Could you check a few things on this model? Use its own coordinates, in mm. Coordinates: 2 decimals unless noted, no trailing zeros. Write each loop counter-clockwise with the first axis right and the second up, starting at its lowest first coordinate (ties: lowest second). Pieces come first, ordered by that corner, then holes.
```python
from build123d import *

# Parameters (mm, degrees)
F0_W           = 80
F0_H           = 44
F1_DEPTH       = 4
F3_D           = 2.5
F3_DEPTH       = 10
F3_CSINK_D     = 5
F3_CSINK_ANGLE = 81
F5_D           = 4
F5_DEPTH       = 10
F7_D           = 5
F7_DEPTH       = 10
F8_W           = 49.9
F8_H           = 3
F8_W_2         = 2
F8_H_2         = 26
F9_DEPTH       = 1


with BuildPart() as f1:
    # F0 (on Top) → F1 (new body)
    with BuildSketch(Plane.XY):
        Rectangle(F0_W, F0_H)
    extrude(amount=F1_DEPTH)

    # F3
    with Locations(Plane.XY.offset(4)):
        with Locations((-35.7, -17.7), (-35.7, 17.7), (35.7, 17.7), (35.7, -17.7)):
            CounterSinkHole(F3_D / 2, F3_CSINK_D / 2, depth=F3_DEPTH, counter_sink_angle=F3_CSINK_ANGLE)

    # F5
    with Locations(Plane.XY.offset(4)):
        with Locations((-18.5, 15), (-4.5, 15), (9.5, 15), (23.5, 15), (-25.5, 7), (-11.5, 7), (2.5, 7), (16.5, 7), (30.5, 7), (-18.5, 0), (-4.5, 0), (9.5, 0), (23.5, 0), (-25.5, -8), (-11.5, -8), (2.5, -8), (16.5, -8), (30.5, -8), (-18.5, -15), (-4.5, -15), (9.5, -15), (23.5, -15)):
            Hole(F5_D / 2, depth=F5_DEPTH)

    # F7
    with Locations(Plane.XY.offset(4)):
        with Locations((31.5, -0.75)):
            Hole(F7_D / 2, depth=F7_DEPTH)

    # F8 (on face) → F9 (join)
    with BuildSketch(Plane(origin=(0, 0, 0), x_dir=(1, 0, 0), z_dir=(0, 0, -1))):
        with Locations((2.5, 20.5)):
            Rectangle(F8_W, F8_H)
        with Locations((2.5, -20.5)):
            Rectangle(F8_W, F8_H)
        with Locations((35.93, 0)):
            Rectangle(F8_W_2, F8_H_2)
        with Locations((-35.93, 0)):
            Rectangle(F8_W_2, F8_H_2)
    extrude(amount=F9_DEPTH)


solid = f1.part
```
1. I want a section at B-B on y = 7. Give the number of separate pieces and of enclosed holes in the cut face, plus the area to 3 significant figures.
Verdict:
separate pieces: 6
enclosed holes: 0
area: 244 mm2
2. Please list where these lines run through material, in increasing order: line 1 along Y through (x, z) = (-35.7, 1); line 2 along Y through (x, z) = (23.5, 1.85); line 3 along Y through (x, z) = (16.5, 3.1).
Verdict:
line 1: y = -22 to -18.95, -16.45 to 16.45, 18.95 to 22
line 2: y = -22 to -17, -13 to -2, 2 to 13, 17 to 22
line 3: y = -22 to -10, -6 to 5, 9 to 22
3. I want a section at D-D on y = -12. Please give me the cut outline in (x, z), plus the area to 3 significant figures.
Verdict:
outline: (-40, 0) - (-36.93, 0) - (-36.93, -1) - (-34.93, -1) - (-34.93, 0) - (34.93, 0) - (34.93, -1) - (36.93, -1) - (36.93, 0) - (40, 0) - (40, 4) - (-40, 4) - close
area: 324 mm2
4. I want a section at A-A on x = 35.7. Please give me the cut outline in (y, z), plus the area to 3 significant figures.
Verdict:
outline: (-22, 0) - (-18.95, 0) - (-18.95, 2.54) - (-20.2, 4) - (-22, 4) - close; (-16.45, 0) - (-13, 0) - (-13, -1) - (13, -1) - (13, 0) - (16.45, 0) - (16.45, 2.54) - (15.2, 4) - (-15.2, 4) - (-16.45, 2.54) - close; (18.95, 0) - (22, 0) - (22, 4) - (20.2, 4) - (18.95, 2.54) - close
area: 178 mm2
5. For pin 1 (3 mm diameter, centred on x = -35.7, y = -17.7, fed in from +Z); pin 2 (1 mm diameter, centred on x = -16.5, y = -12.5, fed in from -Z), each with a flat end and sliding along its axis, tell me the tip position at first contact or that it passes through.
Verdict:
pin 1: stops at z = 2.83
pin 2: stops at z = 0
6. I want a section at C-C on x = 8.5. Please give me the cut outline in (y, z), plus the area to 3 significant figures.
Verdict:
outline: (-22, -1) - (-19, -1) - (-19, 0) - (-16.73, 0) - (-16.73, 4) - (-22, 4) - close; (-13.27, 0) - (-1.73, 0) - (-1.73, 4) - (-13.27, 4) - close; (1.73, 0) - (13.27, 0) - (13.27, 4) - (1.73, 4) - close; (16.73, 0) - (19, 0) - (19, -1) - (22, -1) - (22, 4) - (16.73, 4) - close
area: 140 mm2
7. If we mould it in two halves opening along Y, with no side actions, what happens to faces 1 (the face through (40, 0, 2)), 2 (the face through (34.51, 18.08, 1.25))? For each: pulls with the +Y half, pulls with the -Y half, needs draft (parallel to the pull), parting line crosses it, or undercut.
Verdict:
face 1: needs draft
face 2: undercut
